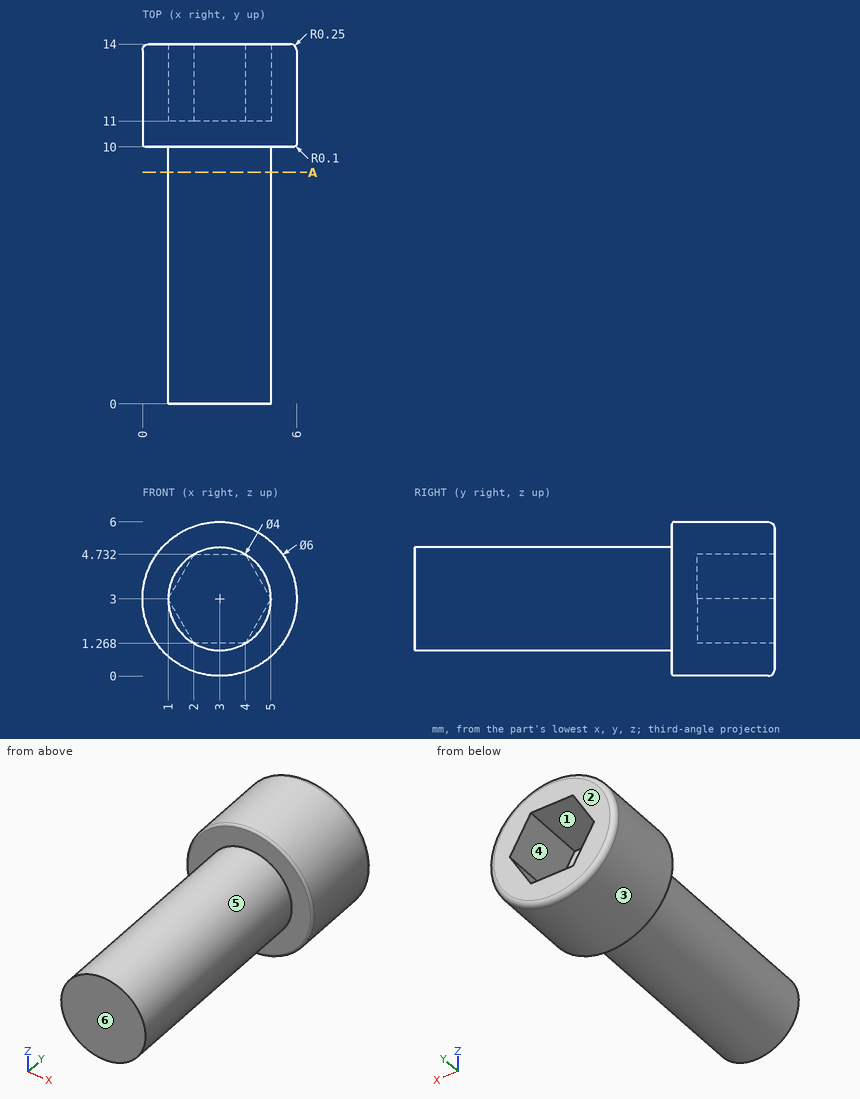
Here's the drawing with two shaded views (mm, measured from the low corner). I have some questions. A direction names the side the tool comes from. Round coordinates to 2 decimals unless told otherwise and drop trailing zeros. Order: outer loops, then holes, each group sorted by start corner. A loop starts at its lowest first (then second) coordinate and runs counter-clockwise, first axis right, second up. Notation, with made-up numbers: (33, 54) -> (51, 54) arc R21 cw to (51, 66) -> close; hole circle Ø1 at (84, 39.25). An arc over 180 degrees is marked (long way). Write each question's results on one line, items separated by ' | '. Start each with the question number.
Item 1: If we section it at A-A, the plane y = 9: Write out the boundary of the cut face in (x, z).
Item 2: Will these pins go through, and if not, where does the flat tip stop? pin 1 (1 mm diameter, centred on x = 3, z = 3, fed in from -Y); pin 2 (3 mm diameter, centred on y = 11.5, z = 5, fed in from -X).
Item 3: Please list where these lines run through material, in increasing order: L1, parallel to Y at x = 1.75, z = 4.75; L2, parallel to X at y = 11.25, z = 3.25; L3, parallel to Z at x = 2, y = 8.5.
Item 4: Thinking about a two-plate mould opening in X: for the marked faces 1, 2 and 3, which applies, +X half, -X half, draft (parallel to the pull), parting line (faces both ways), or undercut?
Item 5: Which directions (+Z, -Z, +X, -X, +Y, -Y) give clear straight access to the entire face, cutting with the end or side of a thin tool? Please do the marked faces 4, 5 and 6.
Results:
1) outline: circle Ø4 at (3, 3)
2) pin 1: stops at y = 0 | pin 2: stops at x = 0.04
3) L1: y = 10 to 14 | L2: x = 0.01 to 1.14, 4.86 to 5.99 | L3: z = 1.27 to 4.73
4) face 1: undercut | face 2: draft | face 3: parting line
5) face 4: +Y | face 5: -Y | face 6: +Z, -Z, +X, -X, -Y
